Build history of the part. All positions in model axes, mm. Round coordinates to 2 decimals unless told otherwise and drop trailing zeros. Loops run counter-clockwise (first coordinate to the right, second up) from the corner with the lowest first, then second, coordinate; pieces in that order, holes last. Notation, with made-up numbers: (38, 81.25) - (79, 81.25) arc R17 ccw to (79, 109.25) - close; hole circle Ø6 at (-38.75, 37). An arc over 180 degrees is marked (long way). Use a Markdown table: item, result.
Autodesk Fusion 360 part; units mm, degrees
cylinder "CylinderPrimitive1" add diameter 8 height 100 placed x (0, 0, -1) y (0, 1, 0) z (1, 0, 0) at (0, 0, 0)
sphere "SpherePrimitive1" add diameter 15 placed x (0, -1, 0) y (0, 0, 1) z (-1, 0, 0) at (0, 0, 0)
sphere "SpherePrimitive2" add diameter 15 placed x (0, 1, 0) y (0, 0, 1) z (1, 0, 0) at (100, 0, 0)
Q1. Cut at D-D, the plane x = 50. List the corners of the cut face in (y, z).
Results found:
| item | result |
|---|---|
| outline | circle Ø8 at (0, 0) |
Q2. Probe line 1 (X direction, y = -4.5, z = -3.25); line 2 (X direction, y = -1.5, z = 6.5); line 3 (Y direction, x = 17.5, z = -3.25). List the from-to ranges inside material, lowest first.
Results found:
| item | result |
|---|---|
| line 1 | x = -5.04 to 5.04, 94.96 to 105.04 |
| line 2 | x = -3.43 to 3.43, 96.57 to 103.43 |
| line 3 | y = -2.33 to 2.33 |
Q3. Cut at C-C, the plane y = -5. List the corners of the cut face in (x, z).
Results found:
| item | result |
|---|---|
| outline | circle Ø11.18 at (0, 0); circle Ø11.18 at (100, 0) |
Q4. Cut at A-A, the plane y = 0. List the corners of the cut face in (x, z).
Results found:
| item | result |
|---|---|
| outline | (6.34, -4) - (93.66, -4) arc R7.5 ccw (long way) to (93.66, 4) - (6.34, 4) arc R7.5 ccw (long way) to start |
Q5. Drop flat-ended pins along their axis: pin 1 (1 mm diameter, centred on x = 41, z = 1.5, fed in from +Y); pin 2 (3 mm diameter, centred on x = 69.5, y = 1, fed in from -Z); pin 3 (3 mm diameter, centred on y = -3, z = -3.5, fed in from +X). Give the stop position or say it passes through.
Results found:
| item | result |
|---|---|
| pin 1 | stops at y = 3.87 |
| pin 2 | stops at z = -4 |
| pin 3 | stops at x = 106.82 |
